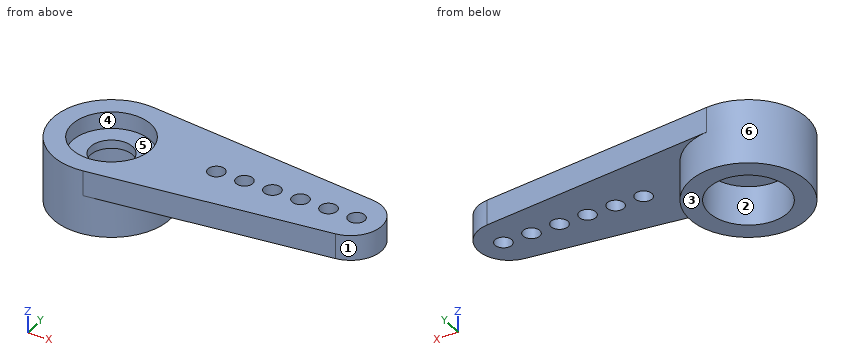
Autodesk Inventor part; units mm, degrees
ref_plane "YZ Plane" through (0, 0, 0) normal (1, 0, 0) x (0, 1, 0)
ref_plane "XZ Plane" through (0, 0, 0) normal (0, 1, 0) x (-1, 0, 0)
ref_plane "XY Plane" through (0, 0, 0) normal (0, 0, 1) x (1, 0, 0)
sketch "Sketch1" plane through (0, 0, 0) normal (0, 0, 1) x (1, 0, 0)
  circle A0 centre (0, 0) radius 3.485
  arc A1 (14.4278, -1.8377) -> (14.4278, 1.8377) centre (14.215, 0) ccw
  line L0 (0.4008, 3.4619) -> (14.4278, 1.8377)
  line L1 (0.4008, -3.4619) -> (14.4278, -1.8377)
  line L2 (0, 0) -> (14.215, 0) construction
  line L3 (16.065, 5.1941) -> (16.065, -8.7582) construction
  line L4 (-3.485, 10.888) -> (-3.485, -12.1485) construction
  circle A2 centre (6.2317, 0) radius 0.5
  circle A3 centre (7.8983, 0) radius 0.5
  circle A4 centre (9.565, 0) radius 0.5
  circle A5 centre (11.2317, 0) radius 0.5
  circle A6 centre (12.8983, 0) radius 0.5
  circle A7 centre (14.565, 0) radius 0.5
  dimension "d1" = 19.55
  dimension "d2" = 1.85
  dimension "d3" = 6.97
  dimension "d4" = 1
  dimension "d7" = 1.6667
  dimension "d12" = 1.5
extrude "Extrusion1" add sketch "Sketch1" along normal blind 1.5
sketch "Sketch2" plane through (0, 0, 1.5) normal (0, 0, 1) x (1, 0, 0)
  arc A0 (0.4008, 3.4619) -> (0.4008, -3.4619) centre (0, 0) ccw
  circle A1 centre (0, 0) radius 1.25
  circle A2 centre (0, 0) radius 2.335
  dimension "d15" = 4.67
  dimension "d16" = 2.5
extrude "Extrusion2" cut sketch "Sketch2" against normal blind 1.5 contours A1 | A2
sketch "Sketch3" plane through (0, 0, 0) normal (0, 0, -1) x (-1, 0, 0)
  circle A0 centre (0, 0) radius 2.335
  circle A1 centre (0, 0) radius 3.485
  line L0 (-0.4008, -3.4619) -> (-14.4278, -1.8377)
extrude "Extrusion3" add sketch "Sketch3" along normal blind 2.33
sketch "Sketch4" plane through (0, 0, 0) normal (0, 0, -1) x (-1, 0, 0)
  circle A0 centre (0, 0) radius 1.25
  circle A1 centre (0, 0) radius 3.485
  circle A2 centre (0, 0) radius 3.485
  dimension "d21" = 2.5
extrude "Extrusion4" add sketch "Sketch4" against normal blind 0.5
properties part number "servo-horn-b"
Input: part model. Units: mm. Frame: model coordinates. Face numbers are marked on the shaded views. A direction names the side the tool comes from. Give positions to 0.01 mm unless a question says otherwise; leave off trailing zeros. Order: outer loops, then holes, each group sorted by start corner. A loop starts at its lowest first (then second) coordinate and runs counter-clockwise, first axis right, second up. Notation, with made-up numbers: (-36.75, 67.25) - (-30.75, 67.25) arc R26 ccw to (-30.75, 99.25) - close; hole circle Ø11 at (64.5, 6.5). An arc over 180 degrees is marked (long way). One line per item, written item: value.
1. Draft query along Y for the marked faces 3, 4, 5 and 6. Return one class per face: released by +Y, released by -Y, zero draft, split by the parting line, or undercut.
Determined:
face 3: zero draft
face 4: undercut
face 5: undercut
face 6: split by the parting line
2. Cut plane C-C, the plane z = 1.25. Output: boundary loops of the cut face in (x, y) (3 decimals), and give its area (3 significant figures).
Determined:
outline: (0.401, -3.462) - (14.428, -1.838) arc R1.85 ccw to (14.428, 1.838) - (0.401, 3.462) arc R3.485 ccw (long way) to start; hole circle Ø4.67 at (0, 0); hole circle Ø1 at (6.232, 0); hole circle Ø1 at (7.898, 0); hole circle Ø1 at (9.565, 0); hole circle Ø1 at (11.232, 0); hole circle Ø1 at (12.898, 0); hole circle Ø1 at (14.565, 0)
area: 79.0 mm2
3. Cut plane D-D, the plane z = 0.2. Output: boundary loops of the cut face in (x, y) (3 decimals), and give its area (3 significant figures).
Determined:
outline: (0.401, -3.462) - (14.428, -1.838) arc R1.85 ccw to (14.428, 1.838) - (0.401, 3.462) arc R3.485 ccw (long way) to start; hole circle Ø2.5 at (0, 0); hole circle Ø1 at (6.232, 0); hole circle Ø1 at (7.898, 0); hole circle Ø1 at (9.565, 0); hole circle Ø1 at (11.232, 0); hole circle Ø1 at (12.898, 0); hole circle Ø1 at (14.565, 0)
area: 91.2 mm2
4. Line query: probe 1 along X at (y, z) = (0, -1.45) (3 decimals); probe 2 along Y at (x, z) = (0, 0.35) (3 decimals); probe 3 along Y at (x, z) = (1, -1.2). Output: solid intervals per line, ascending.
Determined:
probe 1: -3.485 to -2.335, 2.335 to 3.485
probe 2: -3.485 to -1.25, 1.25 to 3.485
probe 3: -3.34 to -2.11, 2.11 to 3.34
5. Cut plane B-B, the plane z = -1.8. Output: boundary loops of the cut face in (x, y) (3 decimals).
Determined:
outline: circle Ø6.97 at (0, 0); hole circle Ø4.67 at (0, 0)
6. Pin query (flat end, axial travel): pin 1 Ø3.5 at (x, y) = (1, -1) entering from +Z; pin 2 Ø3 at (x, y) = (0, 0) entering from +Z; pin 3 Ø3 at (x, y) = (0, 0) entering from -Z. Return the tip coordinate at first contact, or that it passes through.
Determined:
pin 1: z = 1.5
pin 2: z = 0.5
pin 3: z = 0
7. Reachability of the marked faces 1 and 2 from +Z, -Z, +X, -X, +Y, -Y: full face, straight path, thin tool, end or side. Return the list, or none.
Determined:
face 1: +Z, -Z, +X
face 2: -Z
